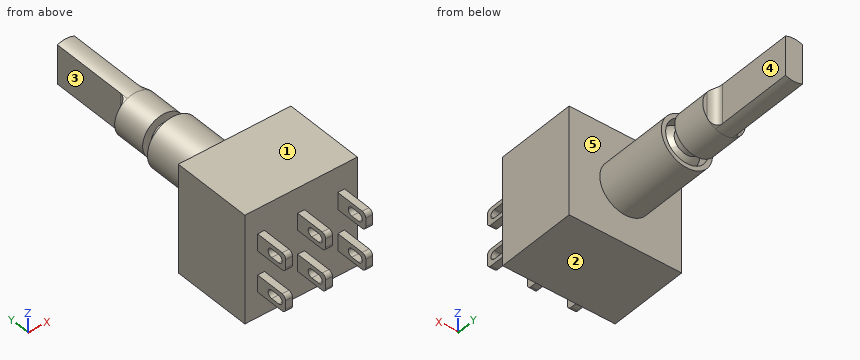
```python
from build123d import *
from build123d.topology import SkipClean

# Parameters (mm, degrees)
SKETCH1_W           = 13.2
SKETCH1_H           = 12.7
BOSS_EXTRUDE1_DEPTH = 9.5
SKETCH2_R           = 3
BOSS_EXTRUDE2_DEPTH = 8.8
SKETCH4_R           = 2.5
CUT_EXTRUDE1_DEPTH  = 2
SKETCH5_R           = 1.5
BOSS_EXTRUDE3_DEPTH = 5
REVOLVE2_ANGLE      = 180
FILLET1_R           = 1
SKETCH6_W           = 0.8
SKETCH6_H           = 2
BOSS_EXTRUDE4_DEPTH = 4
SKETCH7_W           = 1
SKETCH7_H           = 2
CUT_EXTRUDE2_DEPTH  = 26.117773
FILLET2_R           = 0.5
BOSS_EXTRUDE5_START = 5.3
SKETCH8_R           = 2.5
BOSS_EXTRUDE5_DEPTH = 4
BOSS_EXTRUDE6_START = 10
BOSS_EXTRUDE6_DEPTH = 10
FILLET3_R           = 1


# Some blends are built 0.0001 mm under size
with BuildPart() as part:
    # Sketch1 → Boss-Extrude1 (new body)
    with BuildSketch(Plane(origin=(0, 0, 0), x_dir=(1, 0, 0), z_dir=(0, 1, 0))):
        Rectangle(SKETCH1_W, SKETCH1_H)
    extrude(amount=BOSS_EXTRUDE1_DEPTH)

    # Sketch2 → Boss-Extrude2 (add)
    with BuildSketch(Plane(origin=(0, 9.5, 0), x_dir=(1, 0, 0), z_dir=(0, 1, 0))):
        with Locations(Location((0, 0, 0), (0, 0, 270))):
            Circle(SKETCH2_R)
    extrude(amount=BOSS_EXTRUDE2_DEPTH)

    # Sketch4 → Cut-Extrude1 (cut)
    with BuildSketch(Plane(origin=(0, 18.3, 0), x_dir=(1, 0, 0), z_dir=(0, 1, 0))):
        with Locations(Location((0, 0, 0), (0, 0, 270))):
            Circle(SKETCH4_R)
    extrude(amount=-CUT_EXTRUDE1_DEPTH, mode=Mode.SUBTRACT)

    # Sketch5 → Boss-Extrude3 (add)
    with BuildSketch(Plane(origin=(0, 16.3, 0), x_dir=(1, 0, 0), z_dir=(0, 1, 0))):
        with Locations(Location((0, 0, 0), (0, 0, 270))):
            Circle(SKETCH5_R)
    extrude(amount=BOSS_EXTRUDE3_DEPTH)

    # Sketch3 → Revolve2 (revolve)
    with BuildSketch(Plane(origin=(0, 16.3, 0), x_dir=(1, 0, 0), z_dir=(0, 1, 0))):
        with BuildLine():
            Line((0, -2.5), (0, 2.5))
            ThreePointArc((0, 2.5), (-2.5, 0), (0, -2.5))
        make_face()
    revolve(axis=Axis((0, 16.3, 3), (0, 0, -1)), revolution_arc=REVOLVE2_ANGLE)

    # Fillet1
    fillet1_edges = [part.edges().sort_by_distance(p)[0] for p in [
        (0, 21.3, -1.5),
    ]]
    fillet(fillet1_edges, radius=FILLET1_R)

    # Sketch6 → Boss-Extrude4 (add)
    with BuildSketch(Plane.XZ):
        with Locations((-4.7, 2.4)):
            Rectangle(SKETCH6_W, SKETCH6_H)
        with Locations((-4.7, -2.4)):
            Rectangle(SKETCH6_W, SKETCH6_H)
        with Locations((0, -2.4)):
            Rectangle(SKETCH6_W, SKETCH6_H)
        with Locations((0, 2.4)):
            Rectangle(SKETCH6_W, SKETCH6_H)
        with Locations((4.7, 2.4)):
            Rectangle(SKETCH6_W, SKETCH6_H)
        with Locations((4.7, -2.4)):
            Rectangle(SKETCH6_W, SKETCH6_H)
    extrude(amount=BOSS_EXTRUDE4_DEPTH)

    # Sketch7 → Cut-Extrude2 (cut, through all)
    with BuildSketch(Plane.ZY.offset(5.1)):
        with Locations((-2.4, -2.5)):
            Rectangle(SKETCH7_W, SKETCH7_H)
        with Locations((2.4, -2.5)):
            Rectangle(SKETCH7_W, SKETCH7_H)
    extrude(amount=-CUT_EXTRUDE2_DEPTH, mode=Mode.SUBTRACT)

    # Fillet2
    fillet2_edges = [part.edges().sort_by_distance(p)[0] for p in [
        (4.7, -3.5, 2.9),
        (4.7, -3.5, 1.9),
        (4.7, -3.5, -1.9),
        (4.7, -3.5, -2.9),
        (4.7, -1.5, -1.9),
        (4.7, -1.5, 2.9),
        (4.7, -1.5, 1.9),
        (4.7, -1.5, -2.9),
        (0, -1.5, 1.9),
        (0, -1.5, 2.9),
        (0, -3.5, 2.9),
        (0, -3.5, 1.9),
        (0, -3.5, -1.9),
        (0, -3.5, -2.9),
        (0, -1.5, -2.9),
        (0, -1.5, -1.9),
        (-4.7, -3.5, 2.9),
        (-4.7, -1.5, 2.9),
        (-4.7, -3.5, 1.9),
        (-4.7, -1.5, 1.9),
        (-4.7, -1.5, -1.9),
        (-4.7, -1.5, -2.9),
        (-4.7, -3.5, -1.9),
        (-4.7, -3.5, -2.9),
        (0, -4, -1.4),
        (0, -4, -3.4),
        (4.7, -4, -1.4),
        (4.7, -4, -3.4),
        (4.7, -4, 1.4),
        (4.7, -4, 3.4),
        (0, -4, 3.4),
        (0, -4, 1.4),
        (-4.7, -4, 3.4),
        (-4.7, -4, 1.4),
        (-4.7, -4, -1.4),
        (-4.7, -4, -3.4),
    ]]
    fillet(fillet2_edges, radius=FILLET2_R - 0.0001)  # a hair under: the kernel refuses the full size

    # Sketch8 → Boss-Extrude5 (add)
    with BuildSketch(Plane(origin=(0, 18.3, 0), x_dir=(1, 0, 0), z_dir=(0, 1, 0)).offset(BOSS_EXTRUDE5_START)):
        with Locations(Location((0, 0, 0), (0, 0, 270))):
            Circle(SKETCH8_R)
    extrude(amount=-BOSS_EXTRUDE5_DEPTH)

    # Sketch9 → Boss-Extrude6 (add)
    with SkipClean():  # the faces are left unmerged after this step: merging them gives an invalid solid
        with BuildSketch(Plane(origin=(0, 23.6, 0), x_dir=(1, 0, 0), z_dir=(0, 1, 0)).offset(BOSS_EXTRUDE6_START)):
            with BuildLine():
                Line((-1, -2.291288), (-1, 2.291288))
                ThreePointArc((-1, 2.291288), (0, 2.5), (1, 2.291288))
                Line((1, 2.291288), (1, -2.291288))
                ThreePointArc((1, -2.291288), (0, -2.5), (-1, -2.291288))
            make_face()
        extrude(amount=-BOSS_EXTRUDE6_DEPTH)

    # Fillet3
    # the kernel refuses this fillet: 1 mm, written as the material it adds along each edge
    with BuildSketch(Plane(origin=(1, 23.6, -4.791288), x_dir=(1, 0, 0), z_dir=(0, 0, 1))) as fillet3_piece_1_section:
        with BuildLine():
            CenterArc((FILLET3_R, FILLET3_R), FILLET3_R, 180, 90)
            Line((0, FILLET3_R), (0, 0))
            Line((0, 0), (FILLET3_R, 0))
        make_face()
    fillet3_piece_1 = extrude(amount=9.582576, mode=Mode.PRIVATE)
    fillet3_piece_1 = fillet3_piece_1 & Plane(origin=(0, 23.834238, 0), x_dir=(0, 0, 1), z_dir=(0, 1, 0)) * Cylinder(2.5, 24, mode=Mode.PRIVATE)
    add(fillet3_piece_1)
    with BuildSketch(Plane(origin=(-1, 23.6, 4.791288), x_dir=(-1, 0, 0), z_dir=(0, 0, -1))) as fillet3_piece_2_section:
        with BuildLine():
            CenterArc((FILLET3_R, FILLET3_R), FILLET3_R, 180, 90)
            Line((0, FILLET3_R), (0, 0))
            Line((0, 0), (FILLET3_R, 0))
        make_face()
    fillet3_piece_2 = extrude(amount=9.582576, mode=Mode.PRIVATE)
    fillet3_piece_2 = fillet3_piece_2 & Plane(origin=(0, 23.834238, 0), x_dir=(0, 0, 1), z_dir=(0, 1, 0)) * Cylinder(2.5, 24, mode=Mode.PRIVATE)
    add(fillet3_piece_2)


solid = part.part
```
Verification items for the finished model (mm, model axes). Face numbers are marked on the shaded views. A direction names the side the tool comes from. Coordinates: 2 decimals unless noted, no trailing zeros. Write each loop counter-clockwise with the first axis right and the second up, starting at its lowest first coordinate (ties: lowest second). Pieces come first, ordered by that corner, then holes. Notation, with made-up numbers: M -5,-21.5 L 51,-21.5 A28 cw 51,16.5 Z; hole C 85,60 d4. An arc over 180 degrees is marked long. Answer as a JSON object with one key per item and string values. Group by question number.
(1) Cross-section at C-C, the plane y = 12. Record the cut outline in (x, z), and give its area (3 significant figures).
(2) Tool access check on the marked faces 1, 2, 3, 4 and 5. Record the directions out of +Z, -Z, +X, -X, +Y, -Y that give a thin tool (end or side, any length) a straight path to the whole face; none if there is none.
(3) Cross-section at A-A, the plane z = 0. Record the cut outline in (x, y).
(4) Material ranges on line 1 (X direction, y = 17.3, z = 0); line 2 (X direction, y = 17.95, z = 0); line 3 (Y direction, x = -3.5, z = -0.75), recorded low to high.
(5) Cross-section at B-B, the plane x = 0. State how many separate pieces and enclosed holes the cut face has, and give its area (3 significant figures).
(6) Cross-section at D-D, the plane y = 22.5. Record the cut outline in (x, z), and give its area (3 significant figures).
(7) Gauge pin test, flat ends, axial feed: pin 1 (1.6 mm diameter, centred on y = -1.5, z = -3, fed in from -X); pin 2 (1.4 mm diameter, centred on y = 28, z = 0, fed in from -X); pin 3 (1 mm diameter, centred on x = 5, z = 0, fed in from +Y). Record the tip position at first contact, or that the pin passes through.
Reply:
{
 "1": {"outline": "C 0,0 d6", "area": "28.3 mm²"},
 "2": {"face 1": "+Z, +X, -X, +Y, -Y", "face 2": "-Z, +X, -X, +Y, -Y", "face 3": "+Z, -Z, -X, +Y", "face 4": "+Z, -Z, +X, +Y", "face 5": "+Y"},
 "3": {"outline": "M -6.6,0 L 6.6,0 L 6.6,9.5 L 3,9.5 L 3,18.3 L 2.5,18.3 L 2.5,16.3 A2.5 ccw 1.5,18.3 L 1.5,19.6 L 2.5,19.6 L 2.5,23.6 L 2,23.6 A1 cw 1,24.6 L 1,33.6 L -1,33.6 L -1,24.6 A1 cw -2,23.6 L -2.5,23.6 L -2.5,19.6 L -1.5,19.6 L -1.5,18.3 A2.5 ccw -2.5,16.3 L -2.5,18.3 L -3,18.3 L -3,9.5 L -6.6,9.5 Z"},
 "4": {"line 1": "-3 to -2.5, -2.29 to 2.29, 2.5 to 3", "line 2": "-3 to -2.5, -1.88 to 1.88, 2.5 to 3", "line 3": "0 to 9.5"},
 "5": {"separate pieces": "1", "enclosed holes": "2", "area": "258 mm²"},
 "6": {"outline": "C 0,0 d5", "area": "19.6 mm²"},
 "7": {"pin 1": "x = -5.1", "pin 2": "x = -1", "pin 3": "y = 9.5"}
}
